```python
from build123d import *

# Parameters (mm, degrees)
SKETCH1_R               = 2.5
SKETCH1_R_2             = 4
SKETCH1_R_3             = 3
BOSS_EXTRUDE1_DEPTH     = 6
CUT_EXTRUDE1_DEPTH      = 62.10646447
CUT_EXTRUDE1_DEPTH_BACK = 62.10646447
CUT_EXTRUDE2_START      = -2
SKETCH4_R               = 8
CUT_EXTRUDE2_DEPTH      = 2
FILLET1_START           = 4
FILLET1_DEPTH           = 2
FILLET2_R               = 0.5
CUT_EXTRUDE3_DEPTH      = 2


with BuildPart() as part:
    # Sketch1 → Boss-Extrude1 (new body)
    with BuildSketch(Plane.XY):
        with BuildLine():
            Line((19.567567568, 32.405405405), (7.567567568, -2.594594595))
            ThreePointArc((7.567567568, -2.594594595), (3.516422912, -7.185733776), (-2.594594595, -7.567567568))
            Line((-2.594594595, -7.567567568), (-37.594594595, 4.432432432))
            ThreePointArc((-37.594594595, 4.432432432), (-42.984429152, 11.50111011), (-38.516422912, 19.185733776))
            Line((-38.516422912, 19.185733776), (8.483577088, 42.185733776))
            ThreePointArc((8.483577088, 42.185733776), (17.293075573, 40.998612422), (19.567567568, 32.405405405))
        make_face()
        with Locations((-35, 12)):
            Circle(SKETCH1_R, mode=Mode.SUBTRACT)
        Circle(SKETCH1_R_2, mode=Mode.SUBTRACT)
        with Locations((12, 35)):
            Circle(SKETCH1_R_3, mode=Mode.SUBTRACT)
    extrude(amount=BOSS_EXTRUDE1_DEPTH)

    # Sketch2 → Cut-Extrude1 (cut, two sides: drawn at the far end of the back side and taken through both)
    with BuildSketch(Plane.XY.offset(6).offset(-CUT_EXTRUDE1_DEPTH_BACK)):
        with BuildLine():
            Line((-27.3724879, 17.959246424), (-15.522864255, 23.75799842))
            ThreePointArc((-15.522864255, 23.75799842), (-14.377048473, 23.829592256), (-13.516209876, 23.070002633))
            Line((-13.516209876, 23.070002633), (-7.71745788, 11.220378988))
            ThreePointArc((-7.71745788, 11.220378988), (-7.940043134, 9.568598022), (-9.551269449, 9.142130773))
            Line((-9.551269449, 9.142130773), (-27.199645091, 15.193002422))
            ThreePointArc((-27.199645091, 15.193002422), (-28.21023907, 16.518379486), (-27.3724879, 17.959246424))
        make_face()
        with BuildLine():
            Line((-25.675675676, 11.445945946), (-10.540540541, 6.256756757))
            ThreePointArc((-10.540540541, 6.256756757), (-8.986486486, 3.081081081), (-12.162162162, 1.527027027))
            Line((-12.162162162, 1.527027027), (-27.297297297, 6.716216216))
            ThreePointArc((-27.297297297, 6.716216216), (-28.851351351, 9.891891892), (-25.675675676, 11.445945946))
        make_face()
        with BuildLine():
            Line((-9.923342988, 24.828214089), (-4.124590991, 12.978590444))
            ThreePointArc((-4.124590991, 12.978590444), (-2.683724054, 12.140839274), (-1.358346989, 13.151433254))
            Line((-1.358346989, 13.151433254), (4.692524659, 30.799808895))
            ThreePointArc((4.692524659, 30.799808895), (4.26605741, 32.41103521), (2.614276444, 32.633620464))
            Line((2.614276444, 32.633620464), (-9.235347201, 26.834868468))
            ThreePointArc((-9.235347201, 26.834868468), (-9.994936824, 25.974029871), (-9.923342988, 24.828214089))
        make_face()
        with BuildLine():
            Line((6.716216216, 27.297297297), (1.527027027, 12.162162162))
            ThreePointArc((1.527027027, 12.162162162), (3.081081081, 8.986486486), (6.256756757, 10.540540541))
            Line((6.256756757, 10.540540541), (11.445945946, 25.675675676))
            ThreePointArc((11.445945946, 25.675675676), (9.891891892, 28.851351351), (6.716216216, 27.297297297))
        make_face()
    extrude(amount=CUT_EXTRUDE1_DEPTH + CUT_EXTRUDE1_DEPTH_BACK, mode=Mode.SUBTRACT)

    # Sketch4 → Cut-Extrude2 (cut)
    with BuildSketch(Plane.XY.offset(6).offset(CUT_EXTRUDE2_START)):
        Circle(SKETCH4_R)
    extrude(amount=CUT_EXTRUDE2_DEPTH, mode=Mode.SUBTRACT)

    # Fillet1: read off the stored shape, not the designer's step
    # Fillet1 outline → Fillet1 (cut)
    with BuildSketch(Plane.XY.offset(FILLET1_START)):
        with BuildLine():
            ThreePointArc((9.402223, 2.75648375), (8.465816464, 2.080853575), (7.516690715, 2.738496066))
            ThreePointArc((7.516690715, 2.738496066), (7.999635991, 0.076315279), (7.567567568, -2.594594595))
            Line((7.567567568, -2.594594595), (9.402223, 2.75648375))
        make_face()
        with BuildLine():
            ThreePointArc((-2.594594595, -7.567567568), (-4.968729766, -6.269906261), (-6.774532102, -4.255081057))
            ThreePointArc((-6.774532102, -4.255081057), (-6.837610332, -5.40805741), (-7.945672939, -5.732912135))
            Line((-7.945672939, -5.732912135), (-2.594594595, -7.567567568))
        make_face()
    extrude(amount=FILLET1_DEPTH, mode=Mode.SUBTRACT)

    # Fillet2
    fillet2_edges = [part.edges().sort_by_distance(p)[0] for p in [
        (-3.516422912, 7.185733776, 4),
        (8.465816464, 2.080853575, 4),
        (-6.837610332, -5.40805741, 4),
    ]]
    fillet(fillet2_edges, radius=FILLET2_R)

    # Sketch5 → Cut-Extrude3 (cut)
    with BuildSketch(Plane(origin=(0, 0, 0), x_dir=(-1, 0, 0), z_dir=(0, 0, -1))):
        with BuildLine():
            Line((37.594594595, 4.432432432), (32.321369427, 7.778040946))
            ThreePointArc((32.321369427, 7.778040946), (30.00973178, 12.311806181), (32.86775168, 16.522556479))
            Line((32.86775168, 16.522556479), (38.516422912, 19.185733776))
            ThreePointArc((38.516422912, 19.185733776), (42.984429152, 11.50111011), (37.594594595, 4.432432432))
        make_face()
    extrude(amount=-CUT_EXTRUDE3_DEPTH, mode=Mode.SUBTRACT)


solid = part.part
```
The listing builds one solid part. Answer for the finished solid, in the listing's coordinates (mm). A direction names the side the tool comes from. Coordinates: 2 decimals unless noted, no trailing zeros. Order: outer loops, then holes, each group sorted by start corner. A loop starts at its lowest first (then second) coordinate and runs counter-clockwise, first axis right, second up. Notation, with made-up numbers: M -40,68 L -25,68 A26 ccw -25,86 Z; hole C 63,-10 d5. An arc over 180 degrees is marked long. Answer as a JSON object with one key per item and string values. Group by question number.
1. Section C-C on y = 35 is taken. Write down the section's boundary in (x, z).
2. Determine the mould class of faces 4 (the cylindrical face through (-42.975, 11.369, 3.972)), 5 (the flat face through (13.65, 15.15, 2.96)), 6 (the cylindrical face through (-28.87, 9.84, 2.96)), 7 (the cylindrical face through (-6.827, -5.394, 5.239)) for opening direction X: released by +X, released by -X, zero draft, split by the parting line, or undercut.
3. Section A-A on x = -34.5 is taken. Write down the section's boundary in (y, z), then the cut area to 3 significant figures.
4. Flat-ended cylindrical pins translate along their axes: P1, Ø1, axis at y = 25.5, z = 3, coming from the -X side; P2, Ø3, axis at y = 21, z = 1, coming from the +X side; P3, Ø4.5, axis at x = -35, y = 12, coming from the -Z side. Find the tip coordinate at first contact, or state that the pin passes through.
5. A tool of negligible diameter and unlimited length cuts with its end or side. For faces 1 (the cylindrical face through (-30, 12, 1)), 2 (the flat face through (-3.228, 29.775, 2.958)), 3 (the flat face through (-15.345, 30.525, 2.958)), from which of +Z, -Z, +X, -X, +Y, -Y can it reach the whole face along a straight path? Write none if from no direction.
6. Section B-B on z = 3.25 is taken. State how many separate pieces and enclosed holes the cut face has, then the cut area to 3 significant figures.
7. Section D-D on x = 0 is taken. Write down the section's boundary in (y, z).
8. Straight lines are drawn through the part: line 1 (Y direction, x = -14, z = 3); line 2 (Y direction, x = -7, z = 4.25); line 3 (X direction, y = 16, z = 1.75). For each, find the intervals that lie inside material, in ascending order.
Values follow:
{
 "1": {"outline": "M -6.2,0 L 9,0 L 9,6 L -6.2,6 Z; M 15,0 L 20,0 L 20,6 L 15,6 Z"},
 "2": {"face 4": "released by -X", "face 5": "released by +X", "face 6": "undercut", "face 7": "split by the parting line"},
 "3": {"outline": "M 3.37,0 L 6.4,0 L 6.4,2 L 9.55,2 L 9.55,6 L 3.37,6 Z; M 14.45,2 L 17.29,2 L 17.29,0 L 21.15,0 L 21.15,6 L 14.45,6 Z", "area": "65.3 mm2"},
 "4": {"P1": "x = -26.64", "P2": "x = 16.17", "P3": "through"},
 "5": {"face 1": "-Z, -X", "face 2": "+Z, -Z", "face 3": "+Z, -Z, -X, +Y"},
 "6": {"separate pieces": "1", "enclosed holes": "7", "area": "1,280 mm2"},
 "7": {"outline": "M -8,0 L -4,0 L -4,4 L -8,4 Z; M 4,0 L 17.11,0 L 17.11,6 L 8,6 L 8,4.5 A0.5 cw 7.5,4 L 4,4 Z; M 31.35,0 L 38.03,0 L 38.03,6 L 31.35,6 Z"},
 "8": {"line 1": "-3.66 to 2.16, 7.44 to 10.67, 23.64 to 31.18", "line 2": "-5.65 to -3.73, 3.73 to 18.85, 27.93 to 34.61", "line 3": "-32 to -28.08, -10.06 to -5.6, -0.38 to 2.84, 8.13 to 13.94"}
}
